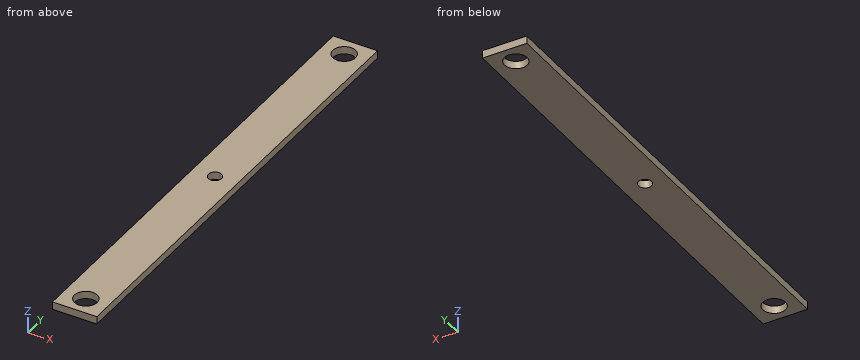
```python
from build123d import *

# Parameters (mm, degrees)
SKETCH1_W           = 11.7
SKETCH1_H           = 125
BOSS_EXTRUDE1_DEPTH = 1
SKETCH2_R           = 3
CUT_EXTRUDE1_DEPTH  = 3
SKETCH3_R           = 1.75
CUT_EXTRUDE2_DEPTH  = 10


with BuildPart() as part:
    # Sketch1 → Boss-Extrude1 (new body, symmetric)
    with BuildSketch(Plane.XY):
        Rectangle(SKETCH1_W, SKETCH1_H)
    extrude(amount=BOSS_EXTRUDE1_DEPTH, both=True)

    # Sketch2 → Cut-Extrude1 (cut, through all)
    with BuildSketch(Plane.XY.offset(1)):
        with Locations((0, 57.5)):
            Circle(SKETCH2_R)
        with Locations((0, -57.5)):
            Circle(SKETCH2_R)
    extrude(amount=-CUT_EXTRUDE1_DEPTH, mode=Mode.SUBTRACT)

    # Sketch3 → Cut-Extrude2 (cut)
    with BuildSketch(Plane.XY.offset(1)):
        Circle(SKETCH3_R)
    extrude(amount=-CUT_EXTRUDE2_DEPTH, mode=Mode.SUBTRACT)


solid = part.part
```
Input: part model. Units: mm. Frame: model coordinates. Coordinates: 2 decimals unless noted, no trailing zeros. Write each loop counter-clockwise with the first axis right and the second up, starting at its lowest first coordinate (ties: lowest second). Pieces come first, ordered by that corner, then holes. Notation, with made-up numbers: (10, -21) - (43, -21) arc R18 cw to (43, -5) - close; hole circle Ø6 at (-19.75, -2.5). An arc over 180 degrees is marked (long way). Put each result on its own line as item: value. Start each with the question number.
1) Cut plane A-A (x = 0). Return the cut outline in (y, z), plus the area to 3 significant figures.
2) Ray query, L1, parallel to Y at x = 0, z = 0.05; L2, parallel to Y at x = 0.75, z = 0.9. Return the intervals inside material, ascending.
3) Cut plane C-C (z = 0.25). Return the cut outline in (x, y).
4) Cut plane D-D (y = -57.5). Return the cut outline in (x, z), plus the area to 3 significant figures.
5) Cut plane B-B (y = 0). Return the cut outline in (x, z), plus the area to 3 significant figures.
Resolved:
1. outline: (-62.5, -1) - (-60.5, -1) - (-60.5, 1) - (-62.5, 1) - close; (-54.5, -1) - (-1.75, -1) - (-1.75, 1) - (-54.5, 1) - close; (1.75, -1) - (54.5, -1) - (54.5, 1) - (1.75, 1) - close; (60.5, -1) - (62.5, -1) - (62.5, 1) - (60.5, 1) - close
1. area: 219 mm2
2. L1: y = -62.5 to -60.5, -54.5 to -1.75, 1.75 to 54.5, 60.5 to 62.5
2. L2: y = -62.5 to -60.4, -54.6 to -1.58, 1.58 to 54.6, 60.4 to 62.5
3. outline: (-5.85, -62.5) - (5.85, -62.5) - (5.85, 62.5) - (-5.85, 62.5) - close; hole circle Ø6 at (0, -57.5); hole circle Ø6 at (0, 57.5); hole circle Ø3.5 at (0, 0)
4. outline: (-5.85, -1) - (-3, -1) - (-3, 1) - (-5.85, 1) - close; (3, -1) - (5.85, -1) - (5.85, 1) - (3, 1) - close
4. area: 11.4 mm2
5. outline: (-5.85, -1) - (-1.75, -1) - (-1.75, 1) - (-5.85, 1) - close; (1.75, -1) - (5.85, -1) - (5.85, 1) - (1.75, 1) - close
5. area: 16.4 mm2
